Source: CAD feature listing. Evaluate the final solid. Frame: model axes, mm. A direction names the side the tool comes from. Give positions to 0.01 mm unless a question says otherwise; leave off trailing zeros. Loops run counter-clockwise (first coordinate to the right, second up) from the corner with the lowest first, then second, coordinate; pieces in that order, holes last. Notation, with made-up numbers: (-6.75, 49.5) - (0.25, 49.5) arc R14 cw to (0.25, 68.5) - close; hole circle Ø10 at (-4, 38). An arc over 180 degrees is marked (long way). Put each result on its own line as item: value.
```python
from build123d import *

# Parameters (mm, degrees)
F0_R     = 8
F0_W     = 15
F0_H     = 2
F1_DEPTH = 3


with BuildPart() as f1:
    # F0 (on Top) → F1 (new body)
    with BuildSketch(Plane.XY):
        Polygon((25.950002, 51.000001), (-24.049998, 51.000001), (-24.049998, 26.000001), (-9.75, 26.000001), (10.25, 26.000001), (25.950002, 26.000001), align=None)
        with Locations((-13.35, 39.000001)):
            Circle(F0_R, mode=Mode.SUBTRACT)
        with Locations((14.549999, 39.000001)):
            Circle(F0_R, mode=Mode.SUBTRACT)
        Polygon((10.25, 26.000001), (-9.75, 26.000001), (-9.75, 14.000001), (-7.05, 14.000001), (7.95, 14.000001), (10.25, 14.000001), align=None)
        with Locations((0.45, 13.000001)):
            Rectangle(F0_W, F0_H)
    extrude(amount=F1_DEPTH)


solid = f1.part
```
1) Material intervals for line 1 along Y through (x, z) = (-13.35, 1.25); line 2 along X through (y, z) = (38, 1.3); line 3 along X through (y, z) = (42.5, 1.2), sorted ascending. Write a range as [from, to].
Check result:
line 1: [26, 31], [47, 51]
line 2: [-24.05, -21.29], [-5.41, 6.61], [22.49, 25.95]
line 3: [-24.05, -20.54], [-6.16, 7.36], [21.74, 25.95]
2) Section query C-C, the plane z = 1.25. Output: boundary loops of the cut face in (x, y).
Check result:
outline: (-24.05, 26) - (-9.75, 26) - (-9.75, 14) - (-7.05, 14) - (-7.05, 12) - (7.95, 12) - (7.95, 14) - (10.25, 14) - (10.25, 26) - (25.95, 26) - (25.95, 51) - (-24.05, 51) - close; hole circle Ø16 at (-13.35, 39); hole circle Ø16 at (14.55, 39)
3) Section query D-D, the plane x = 21. Output: boundary loops of the cut face in (y, z).
Check result:
outline: (26, 0) - (34.27, 0) - (34.27, 3) - (26, 3) - close; (43.73, 0) - (51, 0) - (51, 3) - (43.73, 3) - close
4) Pin query (flat end, axial travel): P1, Ø1.6, axis at y = 13.5, z = 1, coming from the -X side; P2, Ø0.9, axis at x = 16.5, z = 2, coming from the -Y side; P3, Ø21, axis at x = -13.35, y = 39, coming from the -Z side; P4, Ø0.9, axis at y = 22, z = 2, coming from the +X side. Return the tip coordinate at first contact, or that it passes through.
Check result:
P1: x = -9.75
P2: y = 26
P3: z = 0
P4: x = 10.25
5) Section query A-A, the plane x = -13.35. Output: boundary loops of the cut face in (y, z), plus the area to 3 significant figures.
Check result:
outline: (26, 0) - (31, 0) - (31, 3) - (26, 3) - close; (47, 0) - (51, 0) - (51, 3) - (47, 3) - close
area: 27.0 mm²
6) Section query B-B, the plane y = 39. Output: boundary loops of the cut face in (x, z), plus the area to 3 significant figures.
Check result:
outline: (-24.05, 0) - (-21.35, 0) - (-21.35, 3) - (-24.05, 3) - close; (-5.35, 0) - (6.55, 0) - (6.55, 3) - (-5.35, 3) - close; (22.55, 0) - (25.95, 0) - (25.95, 3) - (22.55, 3) - close
area: 54.0 mm²
7) Access query for faces 5 (the flat face through (7.95, 13, 1)), 6 (the flat face through (0, 12, 1)), 7 (the flat face through (-7.05, 13, 1)). Directions: +Z, -Z, +X, -X, +Y, -Y. A direction counts if a zero-diameter tool reaches every point of the face in a straight line with its end or side. Return the directions, or none.
Check result:
face 5: +Z, -Z, +X, -Y
face 6: +Z, -Z, +X, -X, -Y
face 7: +Z, -Z, -X, -Y
8) Mould query, pull axis X, two halves, no side actions, for faces 1 (the flat face through (1, 36, 0)), 2 (the cylindrical face through (18.24, 31.9, 1.48)), 3 (the flat face through (25.95, 38, 1)), 4 (the cylindrical face through (-15.08, 31.19, 1.48)). Classes: pulls with the +X half, pulls with the -X half, needs draft (parallel to the pull), parting line crosses it, or undercut.
Check result:
face 1: needs draft
face 2: undercut
face 3: pulls with the +X half
face 4: undercut
